Build history of the part. All positions in model axes, mm. Give positions to 0.01 mm unless a question says otherwise; leave off trailing zeros. Answer as a JSON object with one key per item and string values. Group by question number.
1. Drill centre lines: line 1 along X through (y, z) = (60, 2.4); line 2 along X through (y, z) = (80.5, 2); line 3 along Y through (x, z) = (-27, 2.3). Where is each one in solid material? Low to high. Write a range as [from, to].
2. Drop flat-ended pins along their axis: pin 1 Ø1.5 at (x, z) = (-150, 2) entering from +Y; pin 2 Ø1.5 at (y, z) = (22.5, 1) entering from +X; pin 3 Ø1.5 at (y, z) = (69.5, 2) entering from -X. Give the stop position or say it passes through.
3. Slice it at A-A (y = 62.5). Give the number of separate pieces and of enclosed holes in the cut face, then the cut area to 3 significant figures.
from build123d import *

# Parameters (mm, degrees)
BOSS_EXTRUDE1_DEPTH = 3
SKETCH2_W           = 2.999999902
SKETCH2_H           = 11.368148841
CUT_EXTRUDE2_DEPTH  = 22
SKETCH4_W           = 3
SKETCH4_H           = 12.91245629
CUT_EXTRUDE3_DEPTH  = 45
SKETCH5_W           = 3
SKETCH5_H           = 17.735525731
CUT_EXTRUDE4_DEPTH  = 38
SKETCH6_W           = 3
SKETCH6_H           = 30.838195809
CUT_EXTRUDE5_DEPTH  = 99
CUT_EXTRUDE6_DEPTH  = 239


with BuildPart() as part:
    # Sketch1 → Boss-Extrude1 (new body)
    with BuildSketch(Plane.XY):
        with BuildLine():
            Line((-200.857104714, 149.999999933), (-200.857104714, 159.999999933))
            Line((-200.857104714, 159.999999933), (-179.730541017, 159.999999933))
            Line((-179.730541017, 159.999999933), (-179.730541017, 149.999999952))
            add(Edge.make_bspline(
                [(-179.730541017, 149.999999952), (-179.435736312, 149.148237058), (-178.129369157, 145.400432959), (-175.809971558, 138.948879894), (-172.785816957, 130.935113712), (-168.767754052, 120.798312408), (-163.776796791, 109.130589637), (-157.847435598, 96.632896439), (-151.989239929, 85.54140938), (-144.288735397, 72.497307518), (-134.900677695, 59.219307644), (-124.086780396, 47.326283664), (-113.706041623, 38.64424455), (-103.59432148, 32.380752321), (-93.477134718, 27.890378411), (-83.091397363, 24.726267775), (-68.685014669, 21.878302713), (-49.516353479, 20.30417739), (-25.106590611, 19.975287666), (-1.8e-08, 20.012356167), (25.106590577, 19.975287666), (49.516353446, 20.304177388), (68.685014637, 21.878302709), (83.091397333, 24.726267767), (93.477134689, 27.8903784), (103.594321452, 32.380752306), (113.706041594, 38.644244529), (124.086780366, 47.326283635), (134.900677664, 59.219307605), (144.288735365, 72.497307468), (151.989239896, 85.541409321), (157.847435565, 96.632896373), (163.776796758, 109.130589562), (168.767754018, 120.798312326), (172.785816923, 130.935113624), (175.809971524, 138.948879801), (178.129369121, 145.400432856), (179.435736274, 149.148236946), (179.730540976, 149.999999832)],
                knots=[0.041921013, 0.041921013, 0.041921013, 0.041921013, 0.044025323, 0.051263016, 0.05850071, 0.065738403, 0.080213789, 0.094689176, 0.109164563, 0.123639949, 0.152590722, 0.181541495, 0.210492269, 0.239443042, 0.268393815, 0.297344588, 0.326295361, 0.384196907, 0.442098454, 0.5, 0.557901546, 0.615803093, 0.673704639, 0.702655412, 0.731606185, 0.760556958, 0.789507731, 0.818458504, 0.847409278, 0.876360051, 0.890835437, 0.905310824, 0.91978621, 0.934261597, 0.94149929, 0.948736984, 0.955974677, 0.958078987, 0.958078987, 0.958078987, 0.958078987], degree=3))
            Line((179.730540976, 149.999999832), (179.730540976, 159.999999832))
            Line((179.730540976, 159.999999832), (200.857104679, 159.999999832))
            Line((200.857104679, 159.999999832), (200.857104679, 149.999999828))
            add(Edge.make_bspline(
                [(-200.857104714, 149.999999933), (-100.428552366, -149.999999904), (-1.8e-08, 149.999999877), (100.428552329, -149.999999851), (200.857104679, 149.999999828)],
                knots=[0.03678763, 0.03678763, 0.03678763, 0.03678763, 0.03678763, 0.96321237, 0.96321237, 0.96321237, 0.96321237, 0.96321237], degree=4))
        make_face()
    extrude(amount=BOSS_EXTRUDE1_DEPTH)

    # Sketch2 → Cut-Extrude2 (cut)
    with BuildSketch(Plane.XY):
        with Locations((-4.4e-08, 15.684087839)):
            Rectangle(SKETCH2_W, SKETCH2_H)
    extrude(amount=CUT_EXTRUDE2_DEPTH, mode=Mode.SUBTRACT)

    # Sketch4 → Cut-Extrude3 (cut)
    with BuildSketch(Plane.XY):
        with Locations((99.999999956, 25.672228128)):
            Rectangle(SKETCH4_W, SKETCH4_H)
    extrude(amount=CUT_EXTRUDE3_DEPTH, mode=Mode.SUBTRACT)

    # Sketch5 → Cut-Extrude4 (cut)
    with BuildSketch(Plane.XY):
        with Locations((-100, 28.083762866)):
            Rectangle(SKETCH5_W, SKETCH5_H)
    extrude(amount=CUT_EXTRUDE4_DEPTH, mode=Mode.SUBTRACT)

    # Sketch6 → Cut-Extrude5 (cut)
    with BuildSketch(Plane.XY):
        with Locations((-150, 72.075097905)):
            Rectangle(SKETCH6_W, SKETCH6_H)
    extrude(amount=CUT_EXTRUDE5_DEPTH, mode=Mode.SUBTRACT)

    # Sketch7 → Cut-Extrude6 (cut)
    with BuildSketch(Plane.XY):
        Polygon((148.499999956, 59.949736331), (148.499999956, 86.674548715), (151.499999956, 86.674548715), (151.499999956, 59.949736331), (151.499999956, 56.949736331), (148.499999956, 56.949736331), align=None)
    extrude(amount=CUT_EXTRUDE6_DEPTH, mode=Mode.SUBTRACT)


solid = part.part
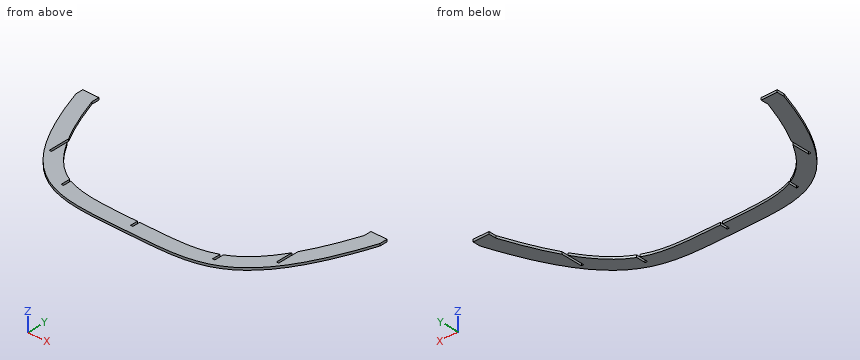
Established:
{
 "1": {"line 1": "x = [-159.74, -151.5], [-148.5, -135.06], [135.06, 148.5], [151.5, 159.74]", "line 2": "x = [-171.91, -151.5], [151.5, 171.91]", "line 3": "y = [0.05, 20.05]"},
 "2": {"pin 1": "stops at y = 56.66", "pin 2": "stops at x = 126.03", "pin 3": "stops at x = -166.16"},
 "3": {"separate pieces": "4", "enclosed holes": "0", "area": "128 mm^2"}
}
